from build123d import *

# Parameters (mm, degrees)
BASPROSKE_W         = 5
BASPROSKE_H         = 22
TOOTHCUT_DEPTH      = 32.511902513
TEETHCUTS_COUNT     = 20
TEETHCUTS_ANGLE     = 342
BORSKE_R            = 2
BORE_DEPTH          = 50.0000508
SKETCH1_W           = 10
SKETCH1_H           = 40
BOSS_EXTRUDE1_DEPTH = 5
CUT_EXTRUDE1_DEPTH  = 61.779759056
SKETCH4_R           = 17.499
BOSS_EXTRUDE2_DEPTH = 5
SKETCH5_R           = 5
CUT_EXTRUDE2_DEPTH  = 5


with BuildPart() as part:
    # BasProSke → Base-Revolve (revolve)
    with BuildSketch(Plane(origin=(0, 0, 0), x_dir=(1, 0, 0), z_dir=(0, 1, 0)), mode=Mode.PRIVATE) as base_revolve_sk:
        with Locations((2.5, 11)):
            Rectangle(BASPROSKE_W, BASPROSKE_H)
    revolve(base_revolve_sk.sketch.rotate(Axis((-10, 0, 0), (1, 0, 0)), 180), axis=Axis((-10, 0, 0), (1, 0, 0)))

    # TooCutSke → ToothCut (cut, through all)
    with BuildSketch(Plane(origin=(0, 0, 0), x_dir=(0, 0, -1), z_dir=(1, 0, 0))):
        with BuildLine():
            ThreePointArc((0.986171591, 17.471189616), (0, 17.499), (-0.986171591, 17.471189616))
            ThreePointArc((-0.986171591, 17.471189616), (-1.626916196, 19.798789858), (-2.932850173, 21.829260982))
            ThreePointArc((-2.932850173, 21.829260982), (0, 22.0254), (2.932850173, 21.829260982))
            ThreePointArc((2.932850173, 21.829260982), (1.626916196, 19.798789858), (0.986171591, 17.471189616))
        make_face()
    toothcut = extrude(amount=TOOTHCUT_DEPTH, mode=Mode.SUBTRACT)

    # TeethCuts: ToothCut ×20 about axis
    teethcuts_axis = Axis((-10, 0, 0), (1, 0, 0))
    for i in range(1, TEETHCUTS_COUNT):
        add(toothcut.rotate(teethcuts_axis, i * TEETHCUTS_ANGLE / (TEETHCUTS_COUNT - 1)), mode=Mode.SUBTRACT)

    # BorSke → Bore (cut, symmetric)
    with BuildSketch(Plane(origin=(0, 0, 0), x_dir=(0, 0, -1), z_dir=(1, 0, 0))):
        with Locations(Location((0, 0, 0), (0, 0, 180))):
            Circle(BORSKE_R)
    extrude(amount=BORE_DEPTH, both=True, mode=Mode.SUBTRACT)

    # Sketch1 → Boss-Extrude1 (add)
    with BuildSketch(Plane.ZY):
        with Locations((0, -36.512502254)):
            Rectangle(SKETCH1_W, SKETCH1_H)
    extrude(amount=-BOSS_EXTRUDE1_DEPTH)

    # Sketch2 → Cut-Extrude1 (cut, through all)
    with BuildSketch(Plane.ZY):
        Polygon((-5, -16.76946633), (-4.460989585, 16.920832513), (-7.792643155, 24.285727196), (-28.634173903, 9.783095201), (-18.213408529, -22.103486404), (-10.962092532, -23.448101291), align=None)
    extrude(amount=-CUT_EXTRUDE1_DEPTH, mode=Mode.SUBTRACT)

    # Sketch4 → Boss-Extrude2 (add)
    with BuildSketch(Plane.ZY):
        Circle(SKETCH4_R)
    extrude(amount=-BOSS_EXTRUDE2_DEPTH)

    # Sketch5 → Cut-Extrude2 (cut)
    with BuildSketch(Plane.ZY):
        Circle(SKETCH5_R)
    extrude(amount=-CUT_EXTRUDE2_DEPTH, mode=Mode.SUBTRACT)


solid = part.part
Build history of the part. All positions in model axes, mm. A direction names the side the tool comes from. Give positions to 0.01 mm unless a question says otherwise; leave off trailing zeros. Order: outer loops, then holes, each group sorted by start corner. A loop starts at its lowest first (then second) coordinate and runs counter-clockwise, first axis right, second up. Notation, with made-up numbers: M 67,28.25 L 121,28.25 A28 ccw 121,66.25 Z; hole C 85,25.5 d9. An arc over 180 degrees is marked long. Put each result on its own line as item: value.
Item 1: Drop a flat-ended pin along its axis: pin 1 Ø1.5 at (x, y) = (3, -33) entering from -Z. Give the stop position or say it passes through.
Results are:
pin 1: z = -5
Item 2: Wall check: probe 1 along Y at (x, z) = (4, 17); probe 2 along Y at (x, z) = (3.6, 18); probe 3 along Z at (x, y) = (4.8, -25.5). Give the ranges that are in metal, low to high.
Results are:
probe 1: -10.33 to -6.7, -4.48 to 4.48, 6.7 to 10.33
probe 2: -10.47 to -7.39, -4.6 to -1.07, 1.07 to 4.6, 7.39 to 10.47
probe 3: -5 to 5
Item 3: Pull direction Z, two halves, no side cores. Call faces 6 (the face through (2.46, 12.97, 15.07)), 7 (the face through (2.46, -4.57, 19.35)), 8 (the face through (2.46, 0.6, -17.49)): +Z half, -Z half, draft (parallel to the pull), parting line (faces both ways), or undercut.
Results are:
face 6: +Z half
face 7: undercut
face 8: -Z half
Item 4: Cut at B-B on y = 0. Write the cut outline in (x, z).
Results are:
outline: M 0,-17.5 L 5,-17.5 L 5,-5 L 0,-5 Z; M 0,5 L 5,5 L 5,17.5 L 0,17.5 Z
Item 5: Cut at A-A on z = 0. Write the cut outline in (x, y), then the cut area to 3 significant figures.
Results are:
outline: M 0,-56.51 L 5,-56.51 L 5,-5 L 0,-5 Z; M 0,5 L 5,5 L 5,17.5 L 0,17.5 Z
area: 320 mm2
Item 6: Cut at C-C on y = -39. Write the cut outline in (x, z).
Results are:
outline: M 0,-5 L 5,-5 L 5,5 L 0,5 Z
Item 7: Cut at D-D on z = -6. Write the cut outline in (x, y).
Results are:
outline: M 0,-16.44 L 5,-16.44 L 5,16.44 L 0,16.44 Z
Item 8: Which spindle directions (+Z, -Z, +X, -X, +Y, -Y) get a long thin tool onto all of the face, cutting with end or side? Do faces 1 (the face through (2.46, 14.17, 10.27)), 2 (the face through (2.465, 15.037, 12.911)), 3 (the face through (2.46, -7.63, 18.29)), 4 (the face through (2.465, -18.341, 7.678)), 5 (the face through (2, -56.513, 0)). Say none if no direction does.
Results are:
face 1: +X, -X
face 2: +X, -X, +Y
face 3: +Z, +X, -X
face 4: +X, -X, -Y
face 5: +Z, -Z, +X, -X, -Y
